from build123d import *
from build123d.topology import SkipClean

# Parameters (mm, degrees)
ESQUISSE1_W                  = 55
ESQUISSE1_H                  = 45
BOSS_EXTRU_1_DEPTH           = 12
ESQUISSE2_R                  = 4.25
ENL_V_MAT_EXTRU_1_DEPTH      = 55.085580333
ENL_V_MAT_EXTRU_2_DEPTH      = 12.25
ENL_V_MAT_EXTRU_2_DEPTH_BACK = 12.25
ESQUISSE3_R                  = 7.75
ESQUISSE9_W                  = 61.062756781
ESQUISSE9_H                  = 12.22812859
ESQUISSE9_W_2                = 59.427147224
ESQUISSE9_H_2                = 8.100161614
ENL_V_MAT_EXTRU_7_DEPTH      = 31
SKETCH1_W                    = 55
SKETCH1_H                    = 36
BOSS_EXTRUDE1_DEPTH          = 5
SKETCH2_R                    = 2.1
CUT_EXTRUDE1_DEPTH           = 38.003378224
SKETCH3_R                    = 4
CUT_EXTRUDE2_DEPTH           = 10
CUT_EXTRUDE3_DEPTH           = 5
SKETCH5_R                    = 2.1
CUT_EXTRUDE4_DEPTH           = 10
BOSS_EXTRUDE4_START          = 2
SKETCH7_R                    = 2.1
BOSS_EXTRUDE4_DEPTH          = 2
SKETCH8_R                    = 2.1
BOSS_EXTRUDE5_DEPTH          = 2
SKETCH9_W                    = 7
SKETCH9_H                    = 3.2
CUT_EXTRUDE6_DEPTH           = 8
ESQUISSE12_R                 = 6
ENL_V_MAT_EXTRU_9_DEPTH      = 12
ESQUISSE13_R                 = 12
ENL_V_MAT_EXTRU_10_DEPTH     = 5


with BuildPart() as part:
    # Esquisse1 → Boss.-Extru.1 (new body)
    with BuildSketch(Plane.XY):
        Rectangle(ESQUISSE1_W, ESQUISSE1_H)
    extrude(amount=BOSS_EXTRU_1_DEPTH)

    # Esquisse2 → Enl_v. mat.-Extru.1 (cut, through all)
    with BuildSketch(Plane(origin=(0, 22.5, 0), x_dir=(1, 0, 0), z_dir=(0, 1, 0))):
        with Locations((-12.5, -12)):
            Circle(ESQUISSE2_R)
        with Locations((12.5, -12)):
            Circle(ESQUISSE2_R)
    extrude(amount=-ENL_V_MAT_EXTRU_1_DEPTH, mode=Mode.SUBTRACT)

    # Esquisse3 → Enl_v. mat.-Extru.2 (cut, two sides: drawn at the far end of the back side and taken through both)
    with BuildSketch(Plane(origin=(0, 0, 0), x_dir=(1, 0, 0), z_dir=(0, 1, 0)).offset(-ENL_V_MAT_EXTRU_2_DEPTH_BACK)):
        with Locations((-12.5, -12)):
            Circle(ESQUISSE3_R)
    extrude(amount=ENL_V_MAT_EXTRU_2_DEPTH + ENL_V_MAT_EXTRU_2_DEPTH_BACK, mode=Mode.SUBTRACT)

    # Esquisse9 → Enl_v. mat.-Extru.7 (cut)
    with BuildSketch(Plane.XY.offset(12)):
        with Locations((-0.389430846, -24.114064295)):
            Rectangle(ESQUISSE9_W, ESQUISSE9_H)
        with Locations((1.674552641, 22.050080807)):
            Rectangle(ESQUISSE9_W_2, ESQUISSE9_H_2)
    extrude(amount=-ENL_V_MAT_EXTRU_7_DEPTH, mode=Mode.SUBTRACT)

    # Sketch1 → Boss-Extrude1 (add)
    with BuildSketch(Plane(origin=(0, 0, 0), x_dir=(-1, 0, 0), z_dir=(0, 0, -1))):
        Rectangle(SKETCH1_W, SKETCH1_H)
    extrude(amount=BOSS_EXTRUDE1_DEPTH)

    # Sketch2 → Cut-Extrude1 (cut, through all)
    with BuildSketch(Plane.XY.offset(12)):
        with Locations((-22.5, 13)):
            Circle(SKETCH2_R)
        with Locations(Location((22.5, 13, 0), (0, 0, 180))):
            Circle(SKETCH2_R)
        with Locations((22.5, -13)):
            Circle(SKETCH2_R)
        with Locations(Location((-22.5, -13, 0), (0, 0, 180))):
            Circle(SKETCH2_R)
    extrude(amount=-CUT_EXTRUDE1_DEPTH, mode=Mode.SUBTRACT)

    # Sketch3 → Cut-Extrude2 (cut)
    with BuildSketch(Plane(origin=(0, 0, -5), x_dir=(-1, 0, 0), z_dir=(0, 0, -1))):
        with Locations((-22.5, 13)):
            Circle(SKETCH3_R)
        with Locations((22.5, 13)):
            Circle(SKETCH3_R)
        with Locations((22.5, -13)):
            Circle(SKETCH3_R)
        with Locations((-22.5, -13)):
            Circle(SKETCH3_R)
    extrude(amount=-CUT_EXTRUDE2_DEPTH, mode=Mode.SUBTRACT)

    # Sketch4 → Cut-Extrude3 (cut)
    with BuildSketch(Plane(origin=(0, 0, -5), x_dir=(-1, 0, 0), z_dir=(0, 0, -1))):
        with BuildLine():
            Line((-18.5, 13), (-18.5, 18))
            Line((-18.5, 18), (-27.5, 18))
            Line((-27.5, 18), (-27.5, 9))
            Line((-27.5, 9), (-22.5, 9))
            ThreePointArc((-22.5, 9), (-25.328427125, 15.828427125), (-18.5, 13))
        make_face()
        with BuildLine():
            Line((-22.5, -9), (-27.5, -9))
            Line((-27.5, -9), (-27.5, -18))
            Line((-27.5, -18), (-18.5, -18))
            Line((-18.5, -18), (-18.5, -13))
            ThreePointArc((-18.5, -13), (-25.328427125, -15.828427125), (-22.5, -9))
        make_face()
        with BuildLine():
            Line((27.5, -18), (27.5, -9))
            Line((27.5, -9), (22.5, -9))
            ThreePointArc((22.5, -9), (25.328427125, -15.828427125), (18.5, -13))
            Line((18.5, -13), (18.5, -18))
            Line((18.5, -18), (27.5, -18))
        make_face()
        with BuildLine():
            Line((27.5, 18), (18.5, 18))
            Line((18.5, 18), (18.5, 13))
            ThreePointArc((18.5, 13), (25.328427125, 15.828427125), (22.5, 9))
            Line((22.5, 9), (27.5, 9))
            Line((27.5, 9), (27.5, 18))
        make_face()
    extrude(amount=-CUT_EXTRUDE3_DEPTH, mode=Mode.SUBTRACT)

    # Sketch5 → Cut-Extrude4 (cut)
    with BuildSketch(Plane(origin=(0, 18, 0), x_dir=(1, 0, 0), z_dir=(0, 1, 0))):
        with Locations(Location((-10, 1, 0), (0, 0, 180))):
            Circle(SKETCH5_R)
        with Locations(Location((10, 1, 0), (0, 0, 180))):
            Circle(SKETCH5_R)
    extrude(amount=-CUT_EXTRUDE4_DEPTH, mode=Mode.SUBTRACT)

    # Sketch7 → Boss-Extrude4 (add)
    with SkipClean():  # the faces are left unmerged after this step: merging them gives an invalid solid
        with BuildSketch(Plane(origin=(0, 18, 0), x_dir=(1, 0, 0), z_dir=(0, 1, 0)).offset(BOSS_EXTRUDE4_START)):
            with BuildLine():
                Line((18.5, 5), (-18.5, 5))
                Line((-18.5, 5), (-18.5, 0))
                Line((-18.5, 0), (-27.5, 0))
                Line((-27.5, 0), (-27.5, -12))
                Line((-27.5, -12), (-16.75, -12))
                ThreePointArc((-16.75, -12), (-12.5, -7.75), (-8.25, -12))
                Line((-8.25, -12), (8.25, -12))
                ThreePointArc((8.25, -12), (12.5, -7.75), (16.75, -12))
                Line((16.75, -12), (27.5, -12))
                Line((27.5, -12), (27.5, 0))
                Line((27.5, 0), (18.5, 0))
                Line((18.5, 0), (18.5, 5))
            make_face()
            with Locations(Location((10, 1, 0), (0, 0, 180))):
                Circle(SKETCH7_R, mode=Mode.SUBTRACT)
            with Locations(Location((-10, 1, 0), (0, 0, 180))):
                Circle(SKETCH7_R, mode=Mode.SUBTRACT)
        extrude(amount=-BOSS_EXTRUDE4_DEPTH)
    add(part.part.scale(1), mode=Mode.REPLACE)  # the faces are merged on a copy

    # Sketch8 → Boss-Extrude5 (add)
    with BuildSketch(Plane.XZ.offset(18)):
        with BuildLine():
            Line((-27.5, 0), (-18.5, 0))
            Line((-18.5, 0), (-18.5, -5))
            Line((-18.5, -5), (18.5, -5))
            Line((18.5, -5), (18.5, 0))
            Line((18.5, 0), (27.5, 0))
            Line((27.5, 0), (27.5, 12))
            Line((27.5, 12), (16.75, 12))
            ThreePointArc((16.75, 12), (12.5, 7.75), (8.25, 12))
            Line((8.25, 12), (-8.25, 12))
            ThreePointArc((-8.25, 12), (-12.5, 7.75), (-16.75, 12))
            Line((-16.75, 12), (-27.5, 12))
            Line((-27.5, 12), (-27.5, 0))
        make_face()
        with Locations(Location((10, -1, 0), (0, 0, 180))):
            Circle(SKETCH8_R, mode=Mode.SUBTRACT)
        with Locations(Location((-10, -1, 0), (0, 0, 180))):
            Circle(SKETCH8_R, mode=Mode.SUBTRACT)
    extrude(amount=BOSS_EXTRUDE5_DEPTH)

    # Sketch9 → Cut-Extrude6 (cut)
    with BuildSketch(Plane(origin=(0, 0, -5), x_dir=(-1, 0, 0), z_dir=(0, 0, -1))):
        with Locations((-10, 14.4)):
            Rectangle(SKETCH9_W, SKETCH9_H)
        with Locations((10, 14.4)):
            Rectangle(SKETCH9_W, SKETCH9_H)
        with Locations((10, -14.4)):
            Rectangle(SKETCH9_W, SKETCH9_H)
        with Locations((-10, -14.4)):
            Rectangle(SKETCH9_W, SKETCH9_H)
    extrude(amount=-CUT_EXTRUDE6_DEPTH, mode=Mode.SUBTRACT)

    # Esquisse12 → Enl_v. mat.-Extru.9 (cut)
    with BuildSketch(Plane(origin=(0, 2, 0), x_dir=(-1, 0, 0), z_dir=(0, -1, 0))):
        with Locations((-12.5, -12)):
            Circle(ESQUISSE12_R)
    extrude(amount=ENL_V_MAT_EXTRU_9_DEPTH, mode=Mode.SUBTRACT)

    # Esquisse13 → Enl_v. mat.-Extru.10 (cut)
    with BuildSketch(Plane(origin=(0, 2, 0), x_dir=(-1, 0, 0), z_dir=(0, -1, 0))):
        with Locations((-12.5, -12)):
            Circle(ESQUISSE13_R)
    extrude(amount=-ENL_V_MAT_EXTRU_10_DEPTH, mode=Mode.SUBTRACT)


solid = part.part
Source: CAD feature listing. Evaluate the final solid. Frame: model axes, mm. A direction names the side the tool comes from. Give positions to 0.01 mm unless a question says otherwise; leave off trailing zeros. Write each loop counter-clockwise with the first axis right and the second up, starting at its lowest first coordinate (ties: lowest second). Pieces come first, ordered by that corner, then holes. Notation, with made-up numbers: M -7,57 L 48,57 A13 ccw 48,74 Z; hole C 46.5,54.5 d9. An arc over 180 degrees is marked long. Return JSON: item names as keys, results as strings. Group by question number.
1) Cut plane A-A, the plane y = 5.5. Output: boundary loops of the cut face in (x, z), plus the area to 3 significant figures.
2) Set-up query: faces 4 (the face through (-24, 17, 0)), 5 (the face through (12.1, -18.99, -1.09)), 6 (the face through (24, 17, 0)), 7 (the face through (-7.9, 18.03, -0.91)). Return all of +Z, -Z, +X, -X, +Y, -Y with unobstructed straight access to the full face (end or side cutting, diameter ignored); none if empty.
3) Pin query (flat end, axial travel): P1, Ø1.5, axis at x = -24.5, z = -2, coming from the -Y side; P2, Ø6.5, axis at x = -22.5, y = -13.5, coming from the -Z side; P3, Ø3.5, axis at x = -10, z = -1, coming from the -Y side. Return the tip coordinate at first contact, or that it passes through.
4) Cut plane C-C, the plane z = -4. Give the number of separate pieces and of enclosed holes in the cut face, plus the area to 3 significant figures.
5) Cut plane D-D, the plane y = -11.5. Output: boundary loops of the cut face in (x, z), plus the area to 3 significant figures.
6) Pull-direction query (Z, two-part tool) for faces 1 (the face through (-27.5, 0, 6)), 2 (the face through (-24, -15, 5)), 3 (the face through (-7.9, 10.43, -0.91)); classes: pulls with the +Z half, pulls with the -Z half, needs draft (parallel to the pull), parting line crosses it, or undercut.
7) Material intervals for line 1 along Y through (x, z) = (-22.5, 10.25); line 2 along X through (y, z) = (13.5, -1.75); line 3 along Y through (x, z) = (-7, 2.5), sorted ascending. Write a range as [from, to].
Recorded:
{
 "1": {"outline": "M -27.5,-5 L 27.5,-5 L 27.5,12 L 24.5,12 A12 cw 0.5,12 L -4.75,12 A7.75 cw -20.25,12 L -27.5,12 Z", "area": "614 mm²"},
 "2": {"face 4": "-Z, -X, +Y", "face 5": "-Y", "face 6": "-Z, +X, +Y", "face 7": "+Y"},
 "3": {"P1": "stops at y = -9", "P2": "stops at z = 5", "P3": "stops at y = -18"},
 "4": {"separate pieces": "1", "enclosed holes": "4", "area": "1,730 mm²"},
 "5": {"outline": "M -27.5,0 L -26.21,0 L -26.21,5 L -23.97,5 L -23.97,12 L -27.5,12 Z; M -21.03,5 L -18.79,5 L -18.79,-5 L 18.79,-5 L 18.79,5 L 21.03,5 L 21.03,12 L 16.75,12 A4.25 cw 8.25,12 L -4.75,12 A7.75 cw -20.25,12 L -21.03,12 Z; M 23.97,5 L 26.21,5 L 26.21,0 L 27.5,0 L 27.5,12 L 23.97,12 Z", "area": "610 mm²"},
 "6": {"face 1": "needs draft", "face 2": "pulls with the -Z half", "face 3": "undercut"},
 "7": {"line 1": "y = [-20, -15.1], [-10.9, 10.9], [15.1, 20]", "line 2": "x = [-18.5, -13.5], [-6.5, 6.5], [13.5, 18.5]", "line 3": "y = [-20, -16], [-12.8, 12.8], [16, 20]"}
}
